from build123d import *

# Parameters (mm, degrees)
SKETCH_1_W          = 258
SKETCH_1_H          = 200
EXTRUDE_1_DEPTH     = 3
SKETCH_2_R          = 3
SKETCH_2_R_2        = 2
SKETCH_2_R_3        = 2.5
SKETCH_2_W          = 30
SKETCH_2_H          = 30
SKETCH_2_W_2        = 50
SKETCH_2_H_2        = 20
CUT_EXTRUDE_2_DEPTH = 3
CHAMFER_2_SIZE      = 2


with BuildPart() as part:
    # 草图1 → 凸台-拉伸1 (new body)
    with BuildSketch(Plane(origin=(0, 0, 0), x_dir=(0, 0, -1), z_dir=(1, 0, 0))):
        Rectangle(SKETCH_1_W, SKETCH_1_H)
    extrude(amount=EXTRUDE_1_DEPTH)

    # 草图2 → 切除-拉伸2 (cut)
    with BuildSketch(Plane(origin=(0, 0, 0), x_dir=(0, 0, -1), z_dir=(1, 0, 0))):
        with Locations((-114, -9)):
            Circle(SKETCH_2_R)
        with Locations((-114, -64)):
            Circle(SKETCH_2_R)
        with Locations(Location((114, -64, 0), (0, 0, 180))):
            Circle(SKETCH_2_R)
        with Locations(Location((114, -9, 0), (0, 0, 180))):
            Circle(SKETCH_2_R)
        with Locations((-32, -18)):
            Circle(SKETCH_2_R_2)
        with Locations(Location((32, -18, 0), (0, 0, 180))):
            Circle(SKETCH_2_R_2)
        with Locations((-42, -18)):
            Circle(SKETCH_2_R_2)
        with Locations(Location((42, -18, 0), (0, 0, 180))):
            Circle(SKETCH_2_R_2)
        with Locations((-75, -87.5)):
            Circle(SKETCH_2_R_3)
        with Locations((-75, 9.5)):
            Circle(SKETCH_2_R_3)
        with Locations(Location((75, -87.5, 0), (0, 0, 180))):
            Circle(SKETCH_2_R_3)
        with Locations(Location((75, 9.5, 0), (0, 0, 180))):
            Circle(SKETCH_2_R_3)
        with Locations((-65, 9.5)):
            Circle(SKETCH_2_R_2)
        with Locations((-65, -15.5)):
            Circle(SKETCH_2_R_2)
        with Locations((-65, -62.5)):
            Circle(SKETCH_2_R_2)
        with Locations((-65, -87.5)):
            Circle(SKETCH_2_R_2)
        with Locations(Location((65, -87.5, 0), (0, 0, 180))):
            Circle(SKETCH_2_R_2)
        with Locations(Location((65, -62.5, 0), (0, 0, 180))):
            Circle(SKETCH_2_R_2)
        with Locations(Location((65, -15.5, 0), (0, 0, 180))):
            Circle(SKETCH_2_R_2)
        with Locations(Location((65, 9.5, 0), (0, 0, 180))):
            Circle(SKETCH_2_R_2)
        with Locations((-114, 55)):
            Circle(SKETCH_2_R_2)
        with Locations((-84, 85)):
            Circle(SKETCH_2_R_2)
        with Locations((0, 85)):
            Circle(SKETCH_2_R_2)
        with Locations(Location((84, 85, 0), (0, 0, 180))):
            Circle(SKETCH_2_R_2)
        with Locations(Location((114, 55, 0), (0, 0, 180))):
            Circle(SKETCH_2_R_2)
        with Locations((114, 85)):
            Rectangle(SKETCH_2_W, SKETCH_2_H)
        with Locations((-114, 85)):
            Rectangle(SKETCH_2_W, SKETCH_2_H)
        with Locations((0, -50)):
            Rectangle(SKETCH_2_W_2, SKETCH_2_H_2)
    extrude(amount=CUT_EXTRUDE_2_DEPTH, mode=Mode.SUBTRACT)

    # 倒角2
    chamfer_2_edges = [part.edges().sort_by_distance(p)[0] for p in [
        (3, 85, 86),
        (3, 85, 2),
        (3, 55, 116),
        (3, 55, -116),
        (3, 85, -86),
    ]]
    chamfer(chamfer_2_edges, length=CHAMFER_2_SIZE)


solid = part.part
Check sheet for the modelled part. Datum: model origin and axes. Units: mm. Coordinates: 2 decimals unless noted, no trailing zeros. Write each loop counter-clockwise with the first axis right and the second up, starting at its lowest first coordinate (ties: lowest second). Pieces come first, ordered by that corner, then holes.
Item 1: Cross-section at B-B on x = 2.5. Count the separate pieces of the cut face and the enclosed holes in it, then the cut area to 3 significant figures.
Numbers:
separate pieces: 1
enclosed holes: 26
area: 48,300 mm2
Item 2: Cross-section at A-A on y = -54.5. Record the boundary of the cut face in (x, z).
Numbers:
outline: (0, -129) - (3, -129) - (3, -25) - (0, -25) - close; (0, 25) - (3, 25) - (3, 129) - (0, 129) - close
Item 3: Depth check by flat-ended pin: pin 1 Ø5 at (y, z) = (85, -84) entering from +X; pin 2 Ø1.5 at (x, z) = (1, -119.5) entering from +Y; pin 3 Ø4.5 at (y, z) = (55, 114) entering from +X. Enter the tip coordinate at first touch or a pass-through.
Numbers:
pin 1: stops at x = 1.5
pin 2: stops at y = 70
pin 3: stops at x = 1.25
Item 4: Scan lines: probe 1 along Y at (x, z) = (1.85, 75); probe 2 along Y at (x, z) = (1.85, -65); probe 3 along Z at (x, y) = (2.4, -53). Record each from-to range of solid material in increasing order.
Numbers:
probe 1: y = -100 to -90, -85 to 7, 12 to 100
probe 2: y = -100 to -89.5, -85.5 to -64.5, -60.5 to -17.5, -13.5 to 7.5, 11.5 to 100
probe 3: z = -129 to -25, 25 to 129
Item 5: Mould release check, pull along Y, two halves, no side actions. Record for faces 1 (the face through (0, 1, 2)), 2 (the face through (1, -85, 75)): released by +Y, released by -Y, zero draft, split by the parting line, or undercut.
Numbers:
face 1: zero draft
face 2: undercut
